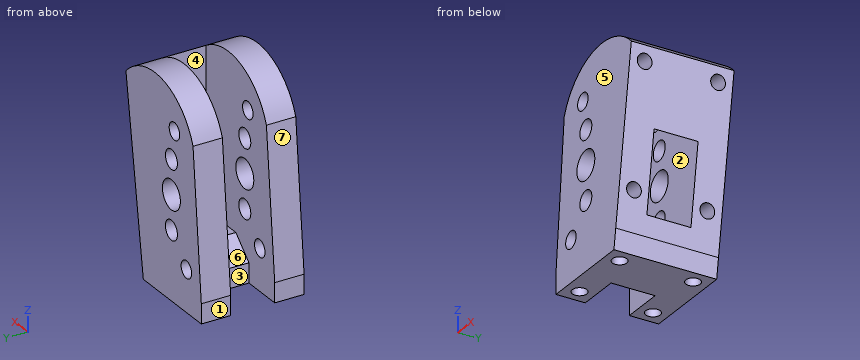
```python
from build123d import *

# Parameters (mm, degrees)
F1_DEPTH    = 10.5
F3_DEPTH    = 4.5
F6_D        = 3.5
F7_T1_DEPTH = 9
F8_R        = 2
F9_DEPTH    = 12.5
F8_R_2      = 3
F11_DEPTH   = 4
F13_DEPTH   = 20
F16_D       = 3
F16_DEPTH   = 8
F16_TIP     = 0.9012909285
F18_D       = 3
F18_DEPTH   = 8
F18_TIP     = 0.9012909285


# Not quite as in the source:
# - a fillet or chamfer that OpenCascade refuses, or shapes differently, is made with other operations: its cross-section is extruded or revolved along the edge and cut away or added


with BuildPart() as f1:
    # F0 (on Front) → F1 (new body, symmetric)
    with BuildSketch(Plane.XZ):
        with BuildLine():
            Line((-10, 0), (10, 0))
            Line((10, 0), (15.209575871, 34.6101187407))
            ThreePointArc((15.209575871, 34.6101187407), (2.6933109979, 38.3883800382), (-7.2260939759, 29.8714821422))
            Line((-7.2260939759, 29.8714821422), (-10, 0))
        make_face()
    extrude(amount=F1_DEPTH, both=True)


with BuildPart() as f3:
    # F2 (on Front) → F3 (new body, symmetric)
    with BuildSketch(Plane.XZ):
        Polygon((-2, 4), (13, 4), (13, 39), (-15, 39), (-15, 0), (-2.371445382, 0), align=None)
    extrude(amount=F3_DEPTH, both=True)


with BuildPart() as f1_1:
    add(f1.part)

    # F4: cut F3
    add(f3.part, mode=Mode.SUBTRACT)

    # F6 (through all)
    with Locations(Plane.XZ.offset(10.5)):
        with Locations((-1, 30), (-5, 4.5)):
            Hole(F6_D / 2)

    # F7: chamfer of 5 on 1 edges, made by hand

    # F7_s2 → F7_t1 (cut)
    with BuildSketch(Plane.XZ.offset(-4.5)):
        Polygon((3, 4), (-2.4623176707, -0.978580357), (-2, 4), align=None)
    extrude(amount=F7_T1_DEPTH, mode=Mode.SUBTRACT)


with BuildPart() as f9:
    # F8 (on Front) → F9 (new body, symmetric)
    with BuildSketch(Plane.XZ):
        with Locations((0, 24)):
            Circle(F8_R)
    extrude(amount=F9_DEPTH, both=True)


with BuildPart() as f9b:
    # F8 (on Front) → F9, piece 2 (new body, symmetric)
    with BuildSketch(Plane.XZ):
        with Locations((0, 17)):
            Circle(F8_R_2)
    extrude(amount=F9_DEPTH, both=True)


with BuildPart() as f9c:
    # F8 (on Front) → F9, piece 3 (new body, symmetric)
    with BuildSketch(Plane.XZ):
        with Locations((0, 10)):
            Circle(F8_R)
    extrude(amount=F9_DEPTH, both=True)


with BuildPart() as f1_2:
    add(f1_1.part)

    # F10: cut F9c, F9b, F9
    add(f9c.part, mode=Mode.SUBTRACT)
    add(f9b.part, mode=Mode.SUBTRACT)
    add(f9.part, mode=Mode.SUBTRACT)

    # F11 (add): a face of the model
    f11_faces = [f1_2.faces().sort_by_distance(p)[0] for p in [
        (1.2885403927, 0, 0),
    ]]
    extrude(f11_faces, amount=F11_DEPTH)


with BuildPart() as f13:
    # F12 (on Front) → F13 (new body, symmetric)
    with BuildSketch(Plane.XZ):
        Polygon((10, -10), (10, 0), (8.4947824334, -10), align=None)
    extrude(amount=F13_DEPTH, both=True)


with BuildPart() as f1_3:
    add(f1_2.part)

    # F14: cut F13
    add(f13.part, mode=Mode.SUBTRACT)

    # F16
    with Locations(Plane(origin=(0, 0, -4), x_dir=(1, 0, 0), z_dir=(0, 0, -1))):
        with Locations((-7, 7.5), (6.3979129734, 7.5), (6.3979129734, -7.5), (-7, -7.5)):
            Hole(F16_D / 2, depth=F16_DEPTH)
            with Locations((0, 0, -(F16_DEPTH + F16_TIP / 2))):  # 118° drill point
                Cone(0, F16_D / 2, F16_TIP, mode=Mode.SUBTRACT)

    # F18
    with Locations(Plane(origin=(9.7784515857, 0, -1.4718697101), x_dir=(0, 1, 0), z_dir=(0.9888605354, 0, -0.1488450249))):
        with Locations((-7.5, 33.4884502488), (7.5, 33.4884502488), (-7.5, 9.4433904486), (7.5, 9.4433904486)):
            Hole(F18_D / 2, depth=F18_DEPTH)
            with Locations((0, 0, -(F18_DEPTH + F18_TIP / 2))):  # 118° drill point
                Cone(0, F18_D / 2, F18_TIP, mode=Mode.SUBTRACT)


solid = f1_3.part
```
Work out the finished part from the listing and answer in its coordinate system (mm). Face numbers are marked on the shaded views. A direction names the side the tool comes from. Give positions to 0.01 mm unless a question says otherwise; leave off trailing zeros. Write each loop counter-clockwise with the first axis right and the second up, starting at its lowest first coordinate (ties: lowest second). Pieces come first, ordered by that corner, then holes. Notation, with made-up numbers: (30, 64) - (86, 64) arc R12 cw to (86, 69) - close; hole circle Ø4 at (20, -5.75). An arc over 180 degrees is marked (long way). Use one line per item in the form item = value.
1. A cutting plane is placed at A-A (y = 5). Write down the section's boundary in (x, z).
Filled in:
outline = (-10, -4) - (9.4, -4) - (15.21, 34.61) arc R13.6 ccw to (-7.23, 29.87) - (-10, 0) - close; hole circle Ø3.5 at (-5, 4.5); hole circle Ø6 at (0, 17); hole circle Ø3.5 at (-1, 30); hole circle Ø4 at (0, 10); hole circle Ø4 at (0, 24)
2. Determine the mould class of the marked faces 4, 5, 6 and 7 for opening direction Y: released by +Y, released by -Y, zero draft, split by the parting line, or undercut.
Filled in:
face_4 = undercut
face_5 = released by -Y
face_6 = undercut
face_7 = zero draft
3. Consider L1, parallel to Y at x = -5.5, z = 22; L2, parallel to Z at x = 0, y = -7.4; L3, parallel to Y at x = -6, z = 2. Determine where each line is inside the solid, lowest interval first.
Filled in:
L1 = -10.5 to -4.5, 4.5 to 10.5
L2 = -4 to 8, 12 to 14, 20 to 22, 26 to 28.56, 31.44 to 37.52
L3 = -10.5 to -8.62, -6.38 to -4.5, 4.5 to 6.38, 8.62 to 10.5
4. For the marked faces 1, 2 and 3, determine the directions among +Z, -Z, +X, -X, +Y, -Y from which every point of the face is accessible in a straight line to the end or side of a thin tool.
Filled in:
face_1 = +Z, -Z, -X, +Y, -Y
face_2 = +Z, -X
face_3 = +Z, -Z, -X
5. Each of these flat-tipped pins is pushed along its axis until it touches: pin 1 Ø2.5 at (x, z) = (0, 10) entering from -Y; pin 2 Ø5 at (x, y) = (7, 5.5) entering from +Z; pin 3 Ø5 at (x, y) = (11.5, 1.5) entering from +Z; pin 4 Ø3 at (y, z) = (2, -1) entering from -X. Where does it stop, or does it pass through?
Filled in:
pin_1 = through
pin_2 = 38.68
pin_3 = 36.43
pin_4 = -1.39
6. A cutting plane is placed at C-C (z = 24). Write down the section's boundary in (x, y).
Filled in:
outline = (-7.77, -10.5) - (-2, -10.5) - (-2, -4.5) - (-7.77, -4.5) - close; (-7.77, 4.5) - (-2, 4.5) - (-2, 10.5) - (-7.77, 10.5) - close; (2, -10.5) - (13.61, -10.5) - (13.61, 10.5) - (2, 10.5) - (2, 4.5) - (13, 4.5) - (13, -4.5) - (2, -4.5) - close
7. A cutting plane is placed at D-D (z = 10). State how many separate pieces and enclosed holes the cut face has, and give its area (3 significant figures).
Filled in:
separate_pieces = 4
enclosed_holes = 2
area = 186 mm^2
8. A cutting plane is placed at B-B (z = 17). Write down the section's boundary in (x, y).
Filled in:
outline = (-8.42, -10.5) - (-3, -10.5) - (-3, -4.5) - (-8.42, -4.5) - close; (-8.42, 4.5) - (-3, 4.5) - (-3, 10.5) - (-8.42, 10.5) - close; (3, -10.5) - (12.56, -10.5) - (12.56, -4.5) - (3, -4.5) - close; (3, 4.5) - (12.56, 4.5) - (12.56, 10.5) - (3, 10.5) - close
